Read the model definition and answer for the solid it produces. Units are mm, in the model's axes. Coordinates: 2 decimals unless noted, no trailing zeros. Write each loop counter-clockwise with the first axis right and the second up, starting at its lowest first coordinate (ties: lowest second). Pieces come first, ordered by that corner, then holes. Notation, with made-up numbers: (-21.5, 50.5) -> (-7.5, 50.5) arc R16 ccw to (-7.5, 60.5) -> close; hole circle Ø3 at (38.25, -29). An arc over 180 degrees is marked (long way). Write item = value, one per line. Start each with the question number.
1) Section C-C (y = 3.25) is taken. Determine the outline of the cut face in (x, z) (3 decimals).
2) Find the intervals of material crossed by line 1 along X through (y, z) = (10.25, 1.5); line 2 along Y through (x, z) = (89, 2.9); line 3 along Y through (x, z) = (128.5, 2.9), in increasing order. Write a range as from..to.
3) Flat-ended cylindrical pins translate along their axes: pin 1 Ø1 at (x, z) = (59.5, 2.5) entering from -Y; pin 2 Ø1.6 at (y, z) = (9, 1.5) entering from +X; pin 3 Ø1.6 at (x, z) = (106, 1.5) entering from -Y. Find the tip coordinate at first contact, or state that the pin passes through.
4) Section D-D (x = 61) is taken. Determine the outline of the cut face in (y, z) (3 decimals).
5) Section B-B (x = 89.5) is taken. Determine the outline of the cut face in (y, z) (1 decimal), plus the area to 3 significant figures.
Solid Edge part; units mm, degrees
sketch "Sketch1" plane through (0, 0, 0) normal (0, 0, 1) x (1, 0, 0)
  line L0 (0, 0) -> (0, 15.875)
  line L1 (0, 15.875) -> (203.2, 15.875)
  line L2 (203.2, 15.875) -> (203.2, 0)
  line L3 (203.2, 0) -> (0, 0)
  dimension "D1" = 203.2
extrude "Protrusion1" add sketch "Sketch1" along normal blind 3.175
sketch "Sketch2" plane through (101.6, 9.525, 3.175) normal (0, 0, 1) x (1, 0, 0)
  line L0 (-25.4, 1.5875) -> (101.6, 1.5875)
  line L1 (101.6, 1.5875) -> (101.6, -1.5875)
  line L2 (101.6, -1.5875) -> (-25.4, -1.5875)
  line L3 (-25.4, -1.5875) -> (-25.4, 1.5875)
  dimension "D1" = 25.4
extrude "Cutout1" cut sketch "Sketch2" against normal through all
sketch "Sketch3" plane through (101.6, 9.525, 3.175) normal (0, 0, 1) x (1, 0, 0)
  line L0 (-101.6, -1.5875) -> (101.6, -9.525)
  line L1 (101.6, -9.525) -> (-101.6, -9.525)
  line L2 (-101.6, -9.525) -> (-101.6, -1.5875)
extrude "Cutout2" cut sketch "Sketch3" against normal through all
sketch "Sketch4" plane through (101.6, 9.525, 3.175) normal (0, 0, 1) x (1, 0, 0)
  line L0 (101.6, 1.5875) -> (50.8, 1.5875)
  line L1 (50.8, 1.5875) -> (-71.12, 6.35)
  line L2 (-71.12, 6.35) -> (101.6, 6.35)
  line L3 (101.6, 6.35) -> (101.6, 1.5875)
extrude "Cutout3" cut sketch "Sketch4" against normal through all
fillet "Round_1" radius 3.175 1 edges at (0, 15.875, 1.5875)
properties material "ABS Plastic, medium impact"
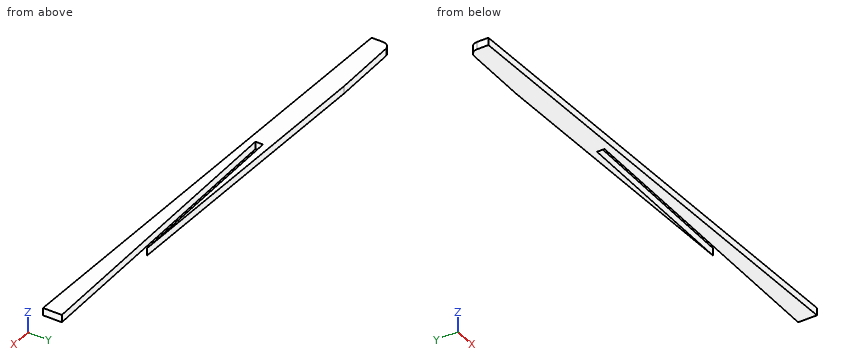
Answer key:
q1.outline = (120, 0) -> (203.2, 0) -> (203.2, 3.175) -> (120, 3.175) -> close
q2.line_1 = 0..76.2
q2.line_2 = 4.46..7.94, 11.11..13.59
q2.line_3 = 2.92..7.94, 11.11..12.05
q3.pin_1 = 5.59
q3.pin_2 = 76.2
q3.pin_3 = 3.77
q4.outline = (5.555, 0) -> (14.683, 0) -> (14.683, 3.175) -> (5.555, 3.175) -> close
q5.outline = (4.4, 0) -> (7.9, 0) -> (7.9, 3.2) -> (4.4, 3.2) -> close; (11.1, 0) -> (13.6, 0) -> (13.6, 3.2) -> (11.1, 3.2) -> close
q5.area = 18.9 mm^2
